Design review of the part built by this model. Coordinates are the model's own, in mm. Face numbers are marked on the shaded views. A direction names the side the tool comes from. Coordinates: 2 decimals unless noted, no trailing zeros. Write each loop counter-clockwise with the first axis right and the second up, starting at its lowest first coordinate (ties: lowest second). Pieces come first, ordered by that corner, then holes.
Q1. For probe 1 along X at (y, z) = (35, 79); probe 2 along X at (y, z) = (6.75, 100); probe 3 along X at (y, z) = (5.5, 40), list the stretches that pass through material, from the lowest coordinate up.
Q2. Mouldability with a two-part tool opening along X and no side actions: class the marked faces 1, 2 and 3 as pulls with the +X half, pulls with the -X half, needs draft (parallel to the pull), parting line crosses it, or undercut.
Q3. Take a section at B-B (z = 51). Give the boundary of the cut face in (x, y).
Q4. Take a section at D-D (y = 4.5). State how many separate pieces and enclosed holes the cut face has, and give its area (3 significant figures).
Q5. Insertion check: pin 1 (3 mm diameter, centred on y = 22, z = 40.5, fed in from -X); pin 2 (10.5 mm diameter, centred on y = 29, z = 64.5, fed in from +X); pin 3 (3 mm diameter, centred on x = -7.5, z = 36.5, fed in from -Y). Each pin has a flat end and moves straight along its axis. Give the tip position at first contact, or say it passes through.
Q6. Take a section at A-A (y = 43.5). Give the boundary of the cut face in (x, z).
Q7. Machinability: for the marked faces 4, 5 and 6, which of the approach directions +Z, -Z, +X, -X, +Y, -Y give a long, thin tool a straight path to every point of the face, cutting with its end or side? Answer none if there is none.
Q8. Take a section at C-C (x = -70). Give the boundary of the cut face in (y, z), and give its area (3 significant figures).
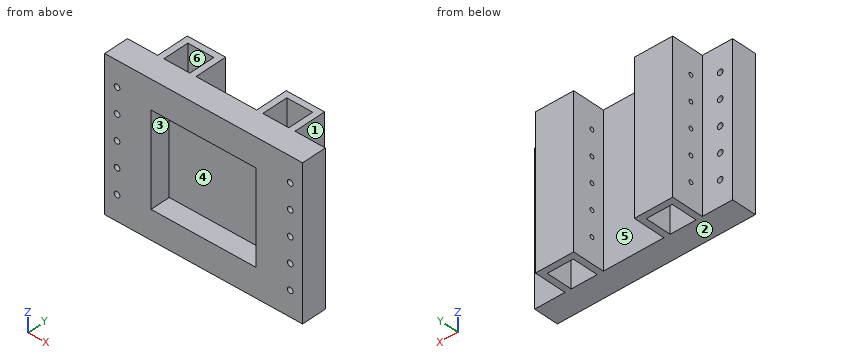
```python
from build123d import *

# Parameters (mm, degrees)
SKETCH_1_W          = 21
SKETCH_1_H          = 21
EXTRUDE_1_DEPTH     = 120
SKETCH_2_W          = 85
SKETCH_2_H          = 74
CUT_EXTRUDE_1_DEPTH = 16
SKETCH_3_R          = 1.65
CUT_EXTRUDE_2_DEPTH = 187.751840687
SKETCH_5_R          = 2.275478237
CUT_EXTRUDE_3_DEPTH = 152.380315761


with BuildPart() as part:
    # 草图1 → 凸台-拉伸1 (new body)
    with BuildSketch(Plane.XY):
        Polygon((-80, 0), (80, 0), (80, 20), (55.5, 20), (55.5, 46), (24.5, 46), (24.5, 20), (-24.5, 20), (-24.5, 46), (-55.5, 46), (-55.5, 20), (-80, 20), align=None)
        with Locations((40, 30.5)):
            Rectangle(SKETCH_1_W, SKETCH_1_H, mode=Mode.SUBTRACT)
        with Locations((-40, 30.5)):
            Rectangle(SKETCH_1_W, SKETCH_1_H, mode=Mode.SUBTRACT)
    extrude(amount=EXTRUDE_1_DEPTH)

    # 草图2 → 切除-拉伸1 (cut)
    with BuildSketch(Plane.XZ):
        with Locations((0, 60)):
            Rectangle(SKETCH_2_W, SKETCH_2_H)
    extrude(amount=-CUT_EXTRUDE_1_DEPTH, mode=Mode.SUBTRACT)

    # 草图3 → 切除-拉伸2 (cut, through all)
    with BuildSketch(Plane.ZY.offset(55.5)):
        with Locations((20, 30)):
            Circle(SKETCH_3_R)
        with Locations((40, 30)):
            Circle(SKETCH_3_R)
        with Locations((60, 30)):
            Circle(SKETCH_3_R)
        with Locations((80, 30)):
            Circle(SKETCH_3_R)
        with Locations((100, 30)):
            Circle(SKETCH_3_R)
    extrude(amount=-CUT_EXTRUDE_2_DEPTH, mode=Mode.SUBTRACT)

    # 草图5 → 切除-拉伸3 (cut, through all)
    with BuildSketch(Plane.XZ):
        with Locations(Location((-70, 100, 0), (0, 0, 270))):
            Circle(SKETCH_5_R)
        with Locations(Location((-70, 80, 0), (0, 0, 270))):
            Circle(SKETCH_5_R)
        with Locations(Location((-70, 60, 0), (0, 0, 270))):
            Circle(SKETCH_5_R)
        with Locations(Location((-70, 40, 0), (0, 0, 270))):
            Circle(SKETCH_5_R)
        with Locations(Location((-70, 20, 0), (0, 0, 270))):
            Circle(SKETCH_5_R)
    cut_extrude_3 = extrude(amount=-CUT_EXTRUDE_3_DEPTH, mode=Mode.SUBTRACT)

    # 镜向1: 切除-拉伸3 across plane
    add(cut_extrude_3.mirror(Plane(origin=(0, 0, 0), x_dir=(0, 0, 1), z_dir=(1, 0, 0))), mode=Mode.SUBTRACT)


solid = part.part
```
Response:
1. probe 1: x = -55.5 to -50.5, -29.5 to -24.5, 24.5 to 29.5, 50.5 to 55.5
1. probe 2: x = -80 to -72.28, -67.72 to 67.72, 72.28 to 80
1. probe 3: x = -80 to -72.28, -67.72 to -42.5, 42.5 to 67.72, 72.28 to 80
2. face 1: pulls with the +X half
2. face 2: needs draft
2. face 3: undercut
3. outline: (-80, 0) - (-42.5, 0) - (-42.5, 16) - (42.5, 16) - (42.5, 0) - (80, 0) - (80, 20) - (55.5, 20) - (55.5, 46) - (24.5, 46) - (24.5, 20) - (-24.5, 20) - (-24.5, 46) - (-55.5, 46) - (-55.5, 20) - (-80, 20) - close; hole (-50.5, 20) - (-29.5, 20) - (-29.5, 41) - (-50.5, 41) - close; hole (29.5, 20) - (50.5, 20) - (50.5, 41) - (29.5, 41) - close
4. separate pieces: 1
4. enclosed holes: 11
4. area: 12,700 mm2
5. pin 1: stops at x = -55.5
5. pin 2: stops at x = 55.5
5. pin 3: stops at y = 16
6. outline: (-55.5, 0) - (-24.5, 0) - (-24.5, 120) - (-55.5, 120) - close; (24.5, 0) - (55.5, 0) - (55.5, 120) - (24.5, 120) - close
7. face 4: -Y
7. face 5: +Z, -Z, +Y
7. face 6: +Z, -Z
8. outline: (0, 0) - (20, 0) - (20, 17.72) - (0, 17.72) - close; (0, 22.28) - (20, 22.28) - (20, 37.72) - (0, 37.72) - close; (0, 42.28) - (20, 42.28) - (20, 57.72) - (0, 57.72) - close; (0, 62.28) - (20, 62.28) - (20, 77.72) - (0, 77.72) - close; (0, 82.28) - (20, 82.28) - (20, 97.72) - (0, 97.72) - close; (0, 102.28) - (20, 102.28) - (20, 120) - (0, 120) - close
8. area: 1,940 mm2
